Here's the drawing with two shaded views (mm, measured from the low corner). I have some questions. Round coordinates to 2 decimals unless told otherwise and drop trailing zeros. Loops run counter-clockwise (first coordinate to the right, second up) from the corner with the lowest first, then second, coordinate; pieces in that order, holes last.
(1) If I drill on line 1 along Y through (x, z) = (8, 1.15); line 2 along X through (y, z) = (7, 0.4), over which ranges is the centre line in solid material (lowest first)?
(2) Thinking about a two-plate mould opening in X: for the marked faces 1, 2 and 3, which applies, released by +X, released by -X, zero draft, split by the parting line, or undercut?
(3) Will these pins go through, and if not, where does the flat tip stop? pin 1 Ø1.5 at (y, z) = (3, 1) entering from -X; pin 2 Ø1 at (x, y) = (7.5, 8.5) entering from -Z; pin 3 Ø1 at (y, z) = (13, 2) entering from -X.
(4) I want a section at C-C on z = 0.9. Write out the boundary of the cut face in (x, y).
(5) I want a section at A-A on x = 8. Write out the boundary of the cut face in (y, z).
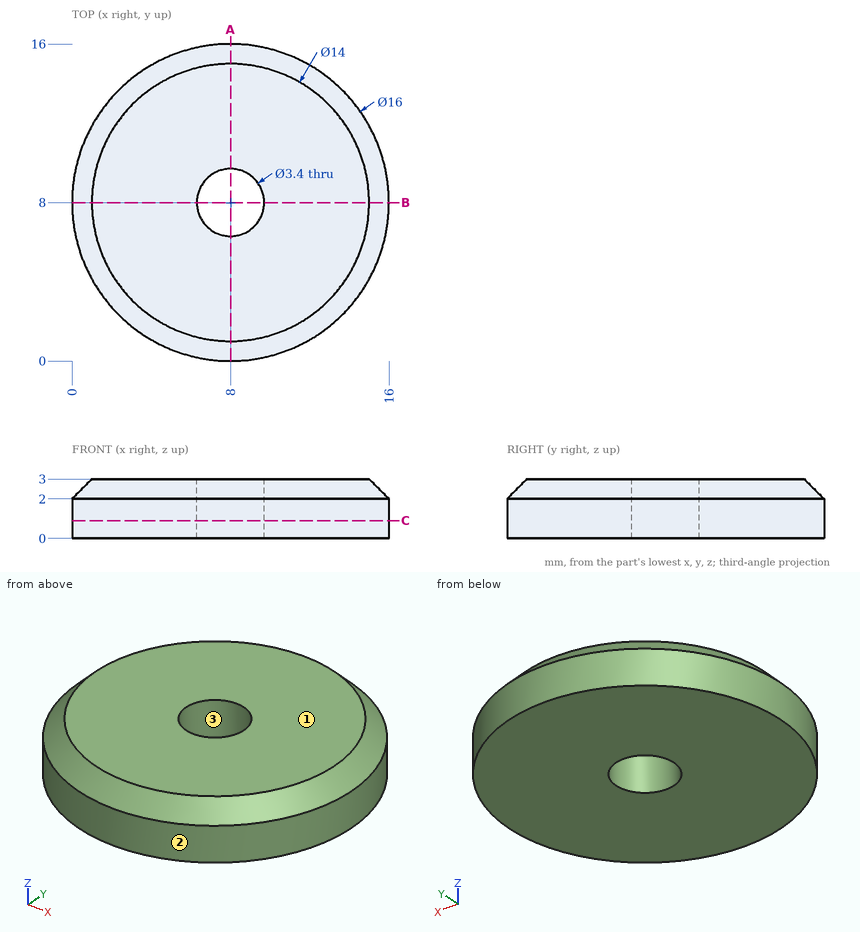
Filled sheet:
1. line 1: y = 0 to 6.3, 9.7 to 16
1. line 2: x = 0.06 to 6.63, 9.37 to 15.94
2. face 1: zero draft
2. face 2: split by the parting line
2. face 3: undercut
3. pin 1: stops at x = 1.22
3. pin 2: passes through
3. pin 3: stops at x = 1.39
4. outline: circle Ø16 at (8, 8); hole circle Ø3.4 at (8, 8)
5. outline: (0, 0) - (6.3, 0) - (6.3, 3) - (1, 3) - (0, 2) - close; (9.7, 0) - (16, 0) - (16, 2) - (15, 3) - (9.7, 3) - close
